Input: part model. Units: mm. Frame: model coordinates. Give positions to 0.01 mm unless a question says otherwise; leave off trailing zeros. Loops run counter-clockwise (first coordinate to the right, second up) from the corner with the lowest first, then second, coordinate; pieces in that order, holes last. Notation, with made-up numbers: (27.5, -27.5) - (74.5, -27.5) arc R26 cw to (74.5, 6.5) - close; hole circle Ø9 at (56, -25.5). An arc over 180 degrees is marked (long way). One line per item, written item: value.
from build123d import *

# Parameters (mm, degrees)
PAD_DEPTH    = 7
SKETCH002_R  = 3.25
POCKET_DEPTH = 2.1


with BuildPart() as part:
    # AdditivePipe: sweep along a path in Sketch001
    with BuildLine(Plane.XY) as additivepipe_path:
        ThreePointArc((0, 3.75), (1.09835, 1.09835), (3.75, 0))
        Line((3.75, 0), (37.75, 0))
        ThreePointArc((37.75, 0), (40.40165, 1.09835), (41.5, 3.75))
        Line((41.5, 3.75), (41.5, 37.75))
        ThreePointArc((41.5, 37.75), (40.40165, 40.40165), (37.75, 41.5))
        Line((37.75, 41.5), (3.75, 41.5))
        ThreePointArc((3.75, 41.5), (1.09835, 40.40165), (0, 37.75))
        Line((0, 37.75), (0, 3.75))
    # Sketch (on Edge2 of Sketch001) → AdditivePipe (sweep)
    with BuildSketch(Plane(origin=(37.75, 0, 0), x_dir=(0, -1, 0), z_dir=(-1, 0, 0))):
        Polygon((-2.95, -7), (-2.15, -6.2), (-2.15, -4.4), (0, -2.25), (0, 0), (-2.95, 0), align=None)
    sweep(path=additivepipe_path.line)

    # Sketch003 (on AdditivePipe) → Pad (new body)
    with BuildSketch(Plane.XY):
        with BuildLine():
            ThreePointArc((3.75, 38.55), (3.184315, 38.315685), (2.95, 37.75))
            Line((2.95, 3.75), (2.95, 37.75))
            ThreePointArc((2.95, 3.75), (3.184315, 3.184315), (3.75, 2.95))
            Line((37.75, 2.95), (3.75, 2.95))
            ThreePointArc((37.75, 2.95), (38.315685, 3.184315), (38.55, 3.75))
            Line((38.55, 37.75), (38.55, 3.75))
            ThreePointArc((38.55, 37.75), (38.315685, 38.315685), (37.75, 38.55))
            Line((3.75, 38.55), (37.75, 38.55))
        make_face()
    extrude(amount=-PAD_DEPTH)

    # Sketch002 (on Face2 of Pad) → Pocket (cut)
    with BuildSketch(Plane(origin=(0, 41.5, -7), x_dir=(1, 0, 0), z_dir=(0, 0, -1))):
        with Locations((7.75, 7.75)):
            Circle(SKETCH002_R)
        with Locations((33.75, 7.75)):
            Circle(SKETCH002_R)
        with Locations((33.75, 33.75)):
            Circle(SKETCH002_R)
        with Locations((7.75, 33.75)):
            Circle(SKETCH002_R)
    extrude(amount=-POCKET_DEPTH, mode=Mode.SUBTRACT)


solid = part.part
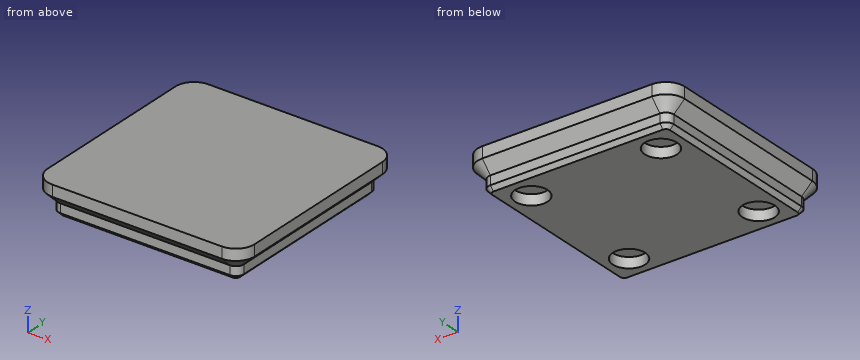
Item 1: Pin query (flat end, axial travel): P1, Ø3, axis at x = 33.5, y = 7, coming from the -Z side; P2, Ø0.9, axis at x = 18.5, z = -5.5, coming from the +Y side; P3, Ø0.9, axis at y = 26.5, z = -5.5, coming from the +X side. Return the tip coordinate at first contact, or that it passes through.
Verdict:
P1: stops at z = -4.9
P2: stops at y = 39.35
P3: stops at x = 39.35
Item 2: Section B-B, the plane y = 33.75. Output: boundary loops of the cut face in (x, z), and give its area (3 significant figures).
Verdict:
outline: (0, -2.25) - (2.15, -4.4) - (2.15, -6.2) - (2.95, -7) - (4.5, -7) - (4.5, -4.9) - (11, -4.9) - (11, -7) - (30.5, -7) - (30.5, -4.9) - (37, -4.9) - (37, -7) - (38.55, -7) - (39.35, -6.2) - (39.35, -4.4) - (41.5, -2.25) - (41.5, 0) - (0, 0) - close
area: 247 mm^2
Item 3: Section D-D, the plane x = 9.5. Output: boundary loops of the cut face in (y, z).
Verdict:
outline: (0, -2.25) - (2.15, -4.4) - (2.15, -6.2) - (2.95, -7) - (5.01, -7) - (5.01, -4.9) - (10.49, -4.9) - (10.49, -7) - (31.01, -7) - (31.01, -4.9) - (36.49, -4.9) - (36.49, -7) - (38.55, -7) - (39.35, -6.2) - (39.35, -4.4) - (41.5, -2.25) - (41.5, 0) - (0, 0) - close
Item 4: Section C-C, the plane z = -3. Output: boundary loops of the cut face in (x, y).
Verdict:
outline: (0.75, 3.75) arc R3 ccw to (3.75, 0.75) - (37.75, 0.75) arc R3 ccw to (40.75, 3.75) - (40.75, 37.75) arc R3 ccw to (37.75, 40.75) - (3.75, 40.75) arc R3 ccw to (0.75, 37.75) - close
Item 5: Material intervals for L1, parallel to X at y = 7.75, z = -5.55, sorted ascending.
Verdict:
L1: x = 2.15 to 4.5, 11 to 30.5, 37 to 39.35
Item 6: Section A-A, the plane z = -5.5. Output: boundary loops of the cut face in (x, y).
Verdict:
outline: (2.15, 3.75) arc R1.6 ccw to (3.75, 2.15) - (37.75, 2.15) arc R1.6 ccw to (39.35, 3.75) - (39.35, 37.75) arc R1.6 ccw to (37.75, 39.35) - (3.75, 39.35) arc R1.6 ccw to (2.15, 37.75) - close; hole circle Ø6.5 at (7.75, 7.75); hole circle Ø6.5 at (7.75, 33.75); hole circle Ø6.5 at (33.75, 7.75); hole circle Ø6.5 at (33.75, 33.75)
